```python
from build123d import *

# Parameters (mm, degrees)
SKETCH1_W           = 54
SKETCH1_H           = 33
BOSS_EXTRUDE1_DEPTH = 3
SKETCH3_W           = 6.5
SKETCH3_H           = 3
BOSS_EXTRUDE2_DEPTH = 21
SKETCH5_R           = 2.15
CUT_EXTRUDE1_DEPTH  = 3
SKETCH6_R           = 1.5
CUT_EXTRUDE2_DEPTH  = 10
BOSS_EXTRUDE3_DEPTH = 6.5
BOSS_EXTRUDE4_DEPTH = 6.5


with BuildPart() as part:
    # Sketch1 → Boss-Extrude1 (new body)
    with BuildSketch(Plane.XY):
        with Locations((7.441119081, -7.107474474)):
            Rectangle(SKETCH1_W, SKETCH1_H)
    extrude(amount=BOSS_EXTRUDE1_DEPTH)

    # Sketch3 → Boss-Extrude2 (add)
    with BuildSketch(Plane.XY.offset(3)):
        with Locations((31.191119081, 5.392525526)):
            Rectangle(SKETCH3_W, SKETCH3_H)
        with Locations((-16.308880919, 5.392525526)):
            Rectangle(SKETCH3_W, SKETCH3_H)
    extrude(amount=BOSS_EXTRUDE2_DEPTH)

    # Sketch5 → Cut-Extrude1 (cut)
    with BuildSketch(Plane(origin=(0, 6.892525526, 0), x_dir=(1, 0, 0), z_dir=(0, 1, 0))):
        with Locations(Location((31.341119081, -18.1, 0), (0, 0, 270))):
            Circle(SKETCH5_R)
        with Locations(Location((31.341119081, -7.9, 0), (0, 0, 270))):
            Circle(SKETCH5_R)
        with Locations(Location((-16.458880919, -18.1, 0), (0, 0, 270))):
            Circle(SKETCH5_R)
        with Locations(Location((-16.458880919, -7.9, 0), (0, 0, 270))):
            Circle(SKETCH5_R)
    extrude(amount=-CUT_EXTRUDE1_DEPTH, mode=Mode.SUBTRACT)

    # Sketch6 → Cut-Extrude2 (cut)
    with BuildSketch(Plane.XY.offset(3)):
        with Locations((31.441119081, -19.607474474)):
            Circle(SKETCH6_R)
        with Locations((-16.558880919, -19.607474474)):
            Circle(SKETCH6_R)
        with Locations((-16.558880919, -6.607474474)):
            Circle(SKETCH6_R)
        with Locations((31.441119081, -6.607474474)):
            Circle(SKETCH6_R)
    extrude(amount=-CUT_EXTRUDE2_DEPTH, mode=Mode.SUBTRACT)

    # Sketch7 → Boss-Extrude3 (add)
    with BuildSketch(Plane(origin=(34.441119081, 0, 0), x_dir=(0, 0, -1), z_dir=(1, 0, 0))):
        Polygon((-5, 3.892525526), (-3, 3.892525526), (-3, 0.892525526), align=None)
    extrude(amount=-BOSS_EXTRUDE3_DEPTH)

    # Sketch8 → Boss-Extrude4 (add)
    with BuildSketch(Plane.ZY.offset(19.558880919)):
        Polygon((5, 3.892525526), (3, 3.892525526), (3, 0.892525526), align=None)
    extrude(amount=-BOSS_EXTRUDE4_DEPTH)


solid = part.part
```
Verification items for the finished model (mm, model axes). A direction names the side the tool comes from. Round coordinates to 2 decimals unless told otherwise and drop trailing zeros. Write each loop counter-clockwise with the first axis right and the second up, starting at its lowest first coordinate (ties: lowest second). Pieces come first, ordered by that corner, then holes. Notation, with made-up numbers: (6.25, -17) - (64.25, -17) arc R29 cw to (64.25, 14) - close; hole circle Ø10 at (-27.5, -38). An arc over 180 degrees is marked (long way). Answer as a JSON object with one key per item and string values. Group by question number.
Q1. Thickness scan on line 1 (X direction, y = 4.7, z = 18.1); line 2 (X direction, y = -20, z = 2.5); line 3 (Z direction, x = 22, y = 3). Record the ranges inside material, lowest first.
Q2. Mould release check, pull along Y, two halves, no side actions. Record for faces 5 (the flat face through (31.237, 2.372, 3.986)), 6 (the flat face through (7, -7, 0)), 7 (the cylindrical face through (-15.173, -7.182, 1.521)): released by +Y, released by -Y, zero draft, split by the parting line, or undercut.
Q3. Section check A-A, the plane z = 7.9. Enter the section's corners in (x, y), plus the area to 3 significant figures.
Q4. Section check D-D, the plane z = 18.5. Enter the section's corners in (x, y), plus the area to 3 significant figures.
Q5. Section check B-B, the plane y = 1.5. Enter the section's corners in (x, z), plus the area to 3 significant figures.
Q6. Go/stop test with flat-tipped pins: pin 1 Ø3 at (x, z) = (32, 19) entering from -Y; pin 2 Ø4 at (y, z) = (-0.5, 5.5) entering from -X; pin 3 Ø7 at (x, z) = (-17.5, 9) entering from +Y. Record where each tip stops, or that it passes through.
Q7. Section check C-C, the plane x = 8.5. Enter the section's corners in (y, z), plus the area to 3 significant figures.
Q8. Tool access check on faces 1 (the flat face through (-13.059, 5, 13)), 2 (the flat face through (-16, 3.893, 14)), 3 (the flat face through (31, 6.893, 13)), 4 (the flat face through (31, 5, 24)). Record the directions out of +Z, -Z, +X, -X, +Y, -Y that give a thin tool (end or side, any length) a straight path to the whole face; none if there is none.
Found:
{
 "1": {"line 1": "x = -19.56 to -18.61, -14.31 to -13.06, 27.94 to 29.19, 33.49 to 34.44", "line 2": "x = -19.56 to -18.01, -15.11 to 29.99, 32.89 to 34.44", "line 3": "z = 0 to 3"},
 "2": {"face 5": "released by -Y", "face 6": "zero draft", "face 7": "undercut"},
 "3": {"outline": "(-19.56, 3.89) - (-18.61, 3.89) - (-18.61, 6.89) - (-19.56, 6.89) - close; (-14.31, 3.89) - (-13.06, 3.89) - (-13.06, 6.89) - (-14.31, 6.89) - close; (27.94, 3.89) - (29.19, 3.89) - (29.19, 6.89) - (27.94, 6.89) - close; (33.49, 3.89) - (34.44, 3.89) - (34.44, 6.89) - (33.49, 6.89) - close", "area": "13.2 mm^2"},
 "4": {"outline": "(-19.56, 3.89) - (-18.57, 3.89) - (-18.57, 6.89) - (-19.56, 6.89) - close; (-14.35, 3.89) - (-13.06, 3.89) - (-13.06, 6.89) - (-14.35, 6.89) - close; (27.94, 3.89) - (29.23, 3.89) - (29.23, 6.89) - (27.94, 6.89) - close; (33.45, 3.89) - (34.44, 3.89) - (34.44, 6.89) - (33.45, 6.89) - close", "area": "13.7 mm^2"},
 "5": {"outline": "(-19.56, 0) - (34.44, 0) - (34.44, 3.4) - (27.94, 3.4) - (27.94, 3) - (-13.06, 3) - (-13.06, 3.4) - (-19.56, 3.4) - close", "area": "167 mm^2"},
 "6": {"pin 1": "stops at y = 3.89", "pin 2": "passes through", "pin 3": "stops at y = 6.89"},
 "7": {"outline": "(-23.61, 0) - (9.39, 0) - (9.39, 3) - (-23.61, 3) - close", "area": "99.0 mm^2"},
 "8": {"face 1": "+Z, +Y, -Y", "face 2": "+Z, +X, -X, -Y", "face 3": "+Z, +X, -X, +Y", "face 4": "+Z, +X, -X, +Y, -Y"}
}
